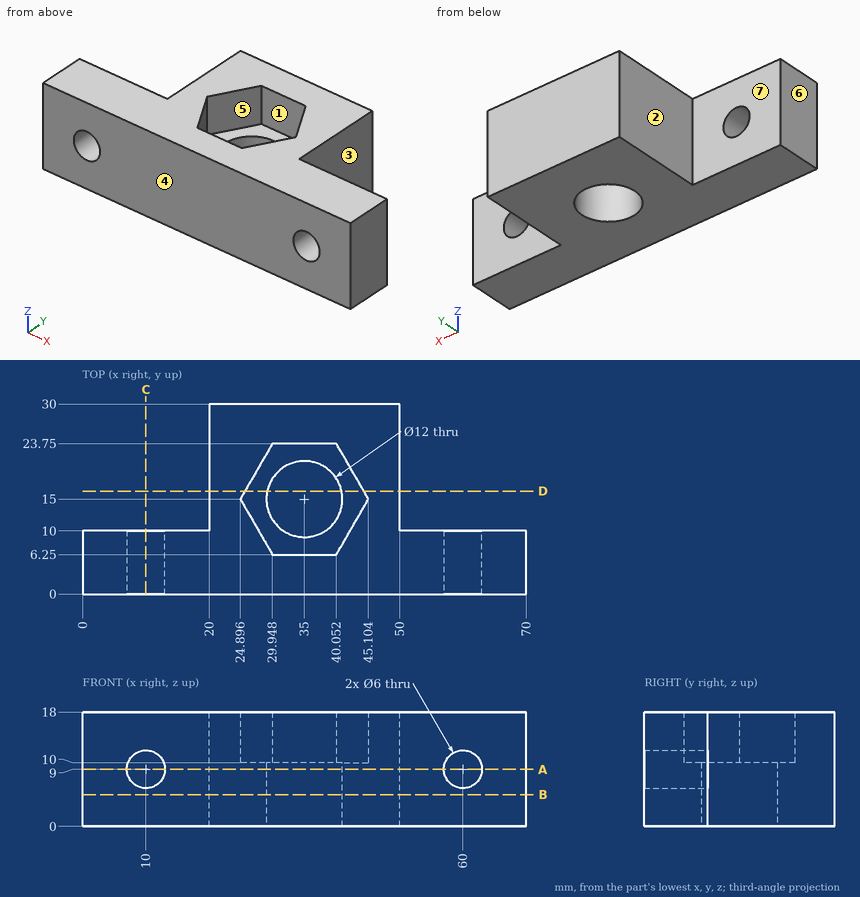
Study the drawing (mm; zero at the part's minimum x, y, z) and answer. A direction names the side the tool comes from. Give positions to 0.01 mm unless a question says otherwise; leave off trailing zeros. Write each loop counter-clockwise with the first axis right and the second up, starting at its lowest first coordinate (ties: lowest second). Pieces come first, ordered by that corner, then holes. Notation, with made-up numbers: (68.5, 89) -> (73.5, 89) arc R12 ccw to (73.5, 98) -> close; hole circle Ø8 at (-21.5, 37). An arc over 180 degrees is marked (long way). Write item = value, one per line. Start each with the question number.
1) The part is cut by section C-C, the plane x = 10. Determine the outline of the cut face in (y, z), and give its area (3 significant figures).
2) Each of these flat-tipped pins is pushed along its axis until it touches: pin 1 (2 mm diameter, centred on x = 17.5, y = 20.5, fed in from -Z); pin 2 (2 mm diameter, centred on x = 42, y = 13, fed in from +Z); pin 3 (5.5 mm diameter, centred on y = 24.5, z = 5.5, fed in from -X); pin 4 (5.5 mm diameter, centred on x = 58, z = 8, fed in from +Y). Where does it stop, or does it pass through?
3) Which of the six approach directions +Z, -Z, +X, -X, +Y, -Y give full straight-line access (tool end or side, diameter ignored) to the marked faces 1, 2, 3 and 4?
4) The part is cut by section D-D, the plane y = 16.25. Determine the outline of the cut face in (x, z).
5) The part is cut by section A-A, the plane z = 9. Determine the outline of the cut face in (x, y), and give its area (3 significant figures).
6) The part is cut by section B-B, the plane z = 5. Determine the outline of the cut face in (x, y), and give its area (3 significant figures).
7) Determine the mould class of the marked faces 5, 6 and 7 for opening direction Y: +Y half, -Y half, draft (parallel to the pull), parting line (faces both ways), or undercut.
8) Straight lines are drawn through the part: line 1 along Z through (x, y) = (60, 8.25); line 2 along Y through (x, z) = (35, 7.25); line 3 along Y through (x, z) = (67, 1.25). For each, find the intervals that lie inside material, in ascending order.
Solutions:
q1.outline = (0, 0) -> (10, 0) -> (10, 6) -> (0, 6) -> close; (0, 12) -> (10, 12) -> (10, 18) -> (0, 18) -> close
q1.area = 120 mm²
q2.pin_1 = through
q2.pin_2 = 10
q2.pin_3 = 20
q2.pin_4 = 10
q3.face_1 = +Z
q3.face_2 = +Z, -Z, -X, +Y
q3.face_3 = +Z, -Z, +X, +Y
q3.face_4 = +Z, -Z, +X, -X, -Y
q4.outline = (20, 0) -> (29.13, 0) -> (29.13, 10) -> (25.62, 10) -> (25.62, 18) -> (20, 18) -> close; (40.87, 0) -> (50, 0) -> (50, 18) -> (44.38, 18) -> (44.38, 10) -> (40.87, 10) -> close
q5.outline = (0, 0) -> (7, 0) -> (7, 10) -> (0, 10) -> close; (13, 0) -> (57, 0) -> (57, 10) -> (50, 10) -> (50, 30) -> (20, 30) -> (20, 10) -> (13, 10) -> close; (63, 0) -> (70, 0) -> (70, 10) -> (63, 10) -> close; hole circle Ø12 at (35, 15)
q5.area = 1,070 mm²
q6.outline = (0, 0) -> (70, 0) -> (70, 10) -> (50, 10) -> (50, 30) -> (20, 30) -> (20, 10) -> (0, 10) -> close; hole circle Ø12 at (35, 15)
q6.area = 1,190 mm²
q7.face_5 = undercut
q7.face_6 = draft
q7.face_7 = +Y half
q8.line_1 = 0 to 6, 12 to 18
q8.line_2 = 0 to 9, 21 to 30
q8.line_3 = 0 to 10
